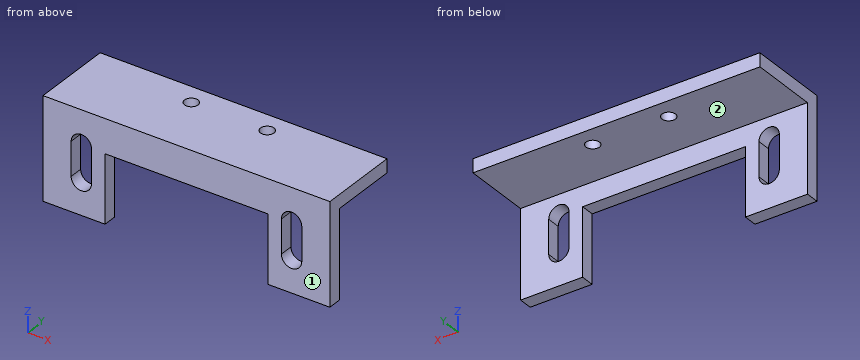
from build123d import *

# Parameters (mm, degrees)
DODANIE_WYCI_GNI_CIE1_DEPTH = 2
SZKIC4_W                    = 42.3
SZKIC4_H                    = 12
SZKIC4_R                    = 1
DODANIE_WYCI_GNI_CIE2_DEPTH = 2


with BuildPart() as part:
    # Szkic1 → Dodanie-wyciągnięcie1 (new body)
    with BuildSketch(Plane(origin=(0, 0, 0), x_dir=(1, 0, 0), z_dir=(0, 1, 0))):
        Polygon((-21.15, 7.5), (-12, 7.5), (-12, -2.5), (12, -2.5), (12, 7.5), (21.15, 7.5), (21.15, -7.5), (-21.15, -7.5), align=None)
        with BuildLine():
            Line((-14, 2.5), (-14, -2.5))
            ThreePointArc((-14, -2.5), (-15.5, -4), (-17, -2.5))
            Line((-17, -2.5), (-17, 2.5))
            ThreePointArc((-17, 2.5), (-15.5, 4), (-14, 2.5))
        make_face(mode=Mode.SUBTRACT)
        with BuildLine():
            Line((17, 2.5), (17, -2.5))
            ThreePointArc((17, -2.5), (15.5, -4), (14, -2.5))
            Line((14, -2.5), (14, 2.5))
            ThreePointArc((14, 2.5), (15.5, 4), (17, 2.5))
        make_face(mode=Mode.SUBTRACT)
    extrude(amount=DODANIE_WYCI_GNI_CIE1_DEPTH)

    # Szkic4 → Dodanie-wyciągnięcie2 (add)
    with BuildSketch(Plane.XY.offset(7.5)):
        with Locations((0, 6)):
            Rectangle(SZKIC4_W, SZKIC4_H)
        with Locations((-5.6, 9)):
            Circle(SZKIC4_R, mode=Mode.SUBTRACT)
        with Locations((5.6, 9)):
            Circle(SZKIC4_R, mode=Mode.SUBTRACT)
    extrude(amount=-DODANIE_WYCI_GNI_CIE2_DEPTH)


solid = part.part
Part model, mm, in its own coordinate system. Face numbers are marked on the shaded views. A direction names the side the tool comes from. Give positions to 0.01 mm unless a question says otherwise; leave off trailing zeros. Loops run counter-clockwise (first coordinate to the right, second up) from the corner with the lowest first, then second, coordinate; pieces in that order, holes last. Notation, with made-up numbers: M 11,17 L 66,17 A24 ccw 66,29 Z; hole C 46,34 d1. An arc over 180 degrees is marked long. Put each result on its own line as item: value. Start each with the question number.
1) Saw through at C-C (y = 1.5). List the corners of the cut face in (x, z), then the cut area to 3 significant figures.
2) 3-axis set-ups, long thin cutter, end or side, ignore diameter. For the marked faces 1 and 2: which of +Z, -Z, +X, -X, +Y, -Y reach the whole face in a straight line?
3) Saw through at D-D (x = 15.5). List the corners of the cut face in (y, z).
4) Flat gauge pins, fed straight in: pin 1 (2 mm diameter, centred on x = 2.5, y = 9, fed in from -Z); pin 2 (1.6 mm diameter, centred on x = -5, y = 1.5, fed in from -Z). Where does each tip first touch, or does it go through?
5) Saw through at A-A (x = -5.6). List the corners of the cut face in (y, z).
6) Probe probe 1 along X at (y, z) = (1, -6.25); probe 2 along Y at (x, z) = (14, -4); probe 3 along Y at (x, z) = (-5.6, 5.9). List the from-to ranges inside material, lowest first.
7) Saw through at B-B (z = -1.75). List the corners of the cut face in (x, y).
Numbers:
1. outline: M -21.15,-7.5 L -12,-7.5 L -12,2.5 L 12,2.5 L 12,-7.5 L 21.15,-7.5 L 21.15,7.5 L -21.15,7.5 Z; hole M -17,-2.5 A1.5 ccw -14,-2.5 L -14,2.5 A1.5 ccw -17,2.5 Z; hole M 14,-2.5 A1.5 ccw 17,-2.5 L 17,2.5 A1.5 ccw 14,2.5 Z
1. area: 350 mm^2
2. face 1: +Z, -Z, +X, -X, -Y
2. face 2: -Z, +X, -X, +Y
3. outline: M 0,-7.5 L 2,-7.5 L 2,-4 L 0,-4 Z; M 0,4 L 2,4 L 2,5.5 L 12,5.5 L 12,7.5 L 0,7.5 Z
4. pin 1: z = 5.5
4. pin 2: z = 2.5
5. outline: M 0,2.5 L 2,2.5 L 2,5.5 L 8,5.5 L 8,7.5 L 0,7.5 Z; M 10,5.5 L 12,5.5 L 12,7.5 L 10,7.5 Z
6. probe 1: -21.15 to -12, 12 to 21.15
6. probe 2: 0 to 2
6. probe 3: 0 to 8, 10 to 12
7. outline: M -21.15,0 L -17,0 L -17,2 L -21.15,2 Z; M -14,0 L -12,0 L -12,2 L -14,2 Z; M 12,0 L 14,0 L 14,2 L 12,2 Z; M 17,0 L 21.15,0 L 21.15,2 L 17,2 Z
